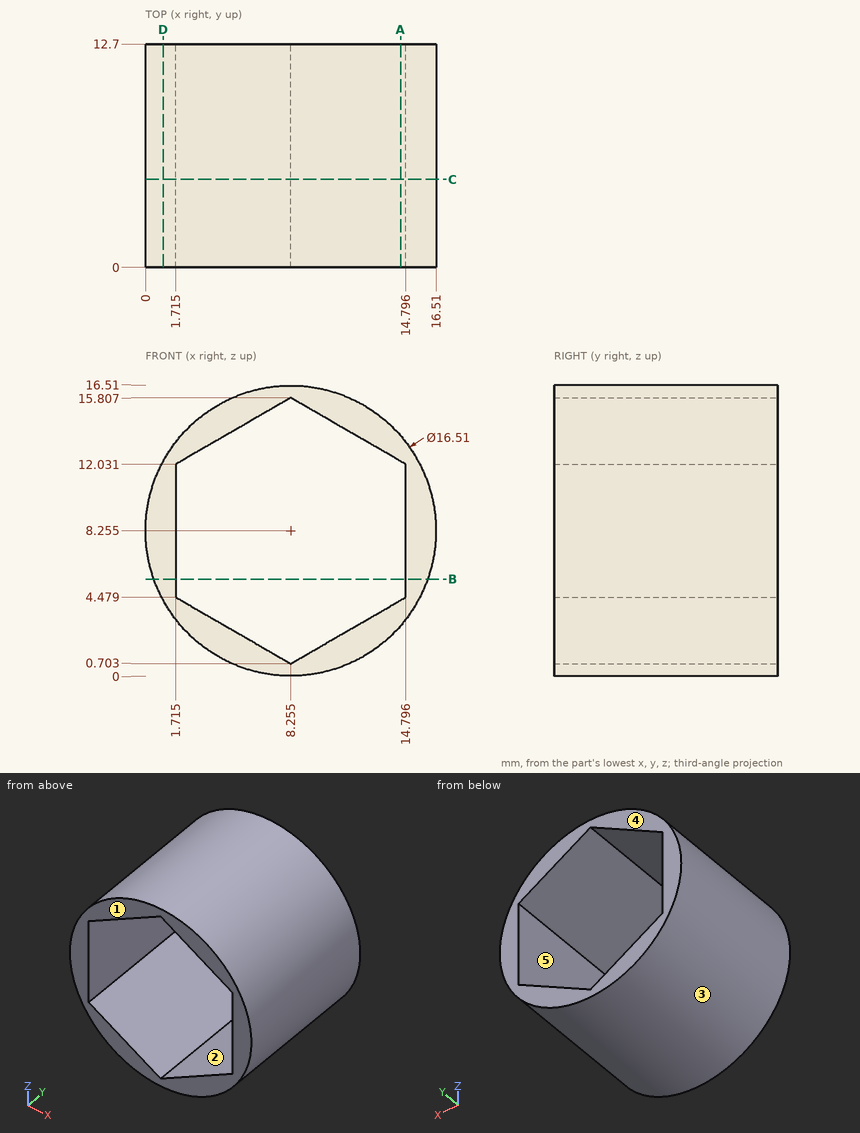
Study the drawing (mm; zero at the part's minimum x, y, z) and answer. A direction names the side the tool comes from. Coordinates: 2 decimals unless noted, no trailing zeros. Write each loop counter-clockwise with the first axis right and the second up, starting at its lowest first coordinate (ties: lowest second). Pieces come first, ordered by that corner, then holes. Notation, with made-up numbers: M 71.5,48.5 L 75.5,48.5 A11 cw 75.5,69.5 Z; hole C 18.5,40 d7. An arc over 180 degrees is marked long. Use one line per item in the form item = value.
Item 1: Find section B-B, the plane z = 5.5. Give the vertices of the cut face in (x, y) (1 decimal).
Model answer:
outline = M 0.5,0 L 1.7,0 L 1.7,12.7 L 0.5,12.7 Z; M 14.8,0 L 16,0 L 16,12.7 L 14.8,12.7 Z
Item 2: Find section A-A, the plane x = 14.5. Give the vertices of the cut face in (y, z).
Model answer:
outline = M 0,2.86 L 12.7,2.86 L 12.7,4.31 L 0,4.31 Z; M 0,12.2 L 12.7,12.2 L 12.7,13.65 L 0,13.65 Z
Item 3: Given P1, Ø4, axis at x = 14.5, y = 9.5, coming from the -Z side (1 decimal); P2, Ø1, axis at x = 12.5, z = 4, coming from the -Y side; P3, Ø2, axis at x = 3.5, y = 5.5, coming from the -Z side, each flat-ended and moving along its own axis, determine where each tip first touches the part or whether it passes through.
Model answer:
P1 = 1.2
P2 = through
P3 = 0.9
Item 4: The mould has two halves that part along Z. Classify the marked faces 1, 2 and 3: released by +Z, released by -Z, zero draft, split by the parting line, or undercut.
Model answer:
face_1 = zero draft
face_2 = undercut
face_3 = split by the parting line
Item 5: For the marked faces 4 and 5, determine the directions among +Z, -Z, +X, -X, +Y, -Y from which every point of the face is accessible in a straight line to the end or side of a thin tool.
Model answer:
face_4 = +Z, -Z, +X, -X, +Y
face_5 = +Y, -Y
Item 6: Find section C-C, the plane y = 5. Give the vertices of the cut face in (x, z) (1 decimal).
Model answer:
outline = C 8.3,8.3 d16.5; hole M 1.7,4.5 L 8.3,0.7 L 14.8,4.5 L 14.8,12 L 8.3,15.8 L 1.7,12 Z
Item 7: Find section D-D, the plane x = 1. Give the vertices of the cut face in (y, z).
Model answer:
outline = M 0,4.32 L 12.7,4.32 L 12.7,12.19 L 0,12.19 Z
Item 8: Find the intervals of material crossed by probe 1 along Z at (x, y) = (6, 6) (1 decimal); probe 2 along Z at (x, y) = (11, 12.25); probe 3 along X at (y, z) = (6.25, 7) (1 decimal), in increasing order.
Model answer:
probe_1 = 0.3 to 2, 14.5 to 16.2
probe_2 = 0.47 to 2.29, 14.22 to 16.04
probe_3 = 0.1 to 1.7, 14.8 to 16.4
